```python
from build123d import *

# Parameters (mm, degrees)
F0_R     = 20
F1_DEPTH = 3.5
F3_R     = 20
F4_DEPTH = 2
F5_W     = 55
F5_H     = 9.110272
F6_DEPTH = 2


with BuildPart() as f1:
    # F0 (on Top) → F1 (new body)
    with BuildSketch(Plane.XY):
        Circle(F0_R)
        Polygon((-12.444864, 12.444864), (-4.555136, 17), (4.555136, 17), (12.444864, 12.444864), (17, 4.555136), (17, -4.555136), (12.444864, -12.444864), (4.555136, -17), (-4.555136, -17), (-12.444864, -12.444864), (-17, -4.555136), (-17, 4.555136), align=None, mode=Mode.SUBTRACT)
    extrude(amount=F1_DEPTH)

    # F3 (on Top) → F4 (join)
    with BuildSketch(Plane.XY):
        Circle(F3_R)
    extrude(amount=F4_DEPTH)

    # F5 (on Top) → F6 (join)
    with BuildSketch(Plane.XY):
        Rectangle(F5_W, F5_H)
    extrude(amount=F6_DEPTH)


solid = f1.part
```
The listing builds one solid part. Answer for the finished solid, in the listing's coordinates (mm). A direction names the side the tool comes from. Give positions to 0.01 mm unless a question says otherwise; leave off trailing zeros. Write each loop counter-clockwise with the first axis right and the second up, starting at its lowest first coordinate (ties: lowest second). Pieces come first, ordered by that corner, then holes. Notation, with made-up numbers: (-3.75, 31) - (2.25, 31) arc R16 ccw to (2.25, 56) - close; hole circle Ø10 at (8.25, 74). An arc over 180 degrees is marked (long way). Use one line per item in the form item = value. Start each with the question number.
1) A tool of negligible diameter and unlimited length cuts with its end or side. For faces 1 (the face through (0, 17, 3)), 2 (the face through (23, 4.555, 1)), 3 (the face through (-27.5, 0, 1)), 4 (the face through (0, 0, 0)), 5 (the face through (-24, -4.555, 1)), from which of +Z, -Z, +X, -X, +Y, -Y can it reach the whole face along a straight path? Write none if from no direction.
2) Consider line 1 along Y through (x, z) = (-0.5, 3); line 2 along Z through (x, y) = (-21.5, 3.5); line 3 along Y through (x, z) = (-15, 2.3). Determine where each line is inside the solid, lowest interval first. Write a range as from..to.
3) Find section C-C on x = 0. Determine the outline of the cut face in (y, z).
4) Find section B-B on y = 0. Determine the outline of the cut face in (x, z), plus the area to 3 significant figures.
5) Flat-ended cylindrical pins translate along their axes: pin 1 Ø1.2 at (y, z) = (0, 2.5) entering from -X; pin 2 Ø2 at (x, z) = (24.5, 1.5) entering from -Y; pin 3 Ø1.6 at (x, z) = (22, 1) entering from +Y; pin 4 Ø17 at (x, y) = (-7, 0.5) entering from +Z. Find the tip coordinate at first contact, or state that the pin passes through.
6) Find section D-D on y = 8. Determine the outline of the cut face in (x, z).
7) Find section A-A on z = 2.85. Determine the outline of the cut face in (x, y).
8) The mould has two halves that part along Y. Classify faces 6 (the face through (-24, 4.555, 1)), 7 (the face through (23, -4.555, 1)), 8 (the face through (14.69, 8.56, 2.74)): pulls with the +Y half, pulls with the -Y half, needs draft (parallel to the pull), parting line crosses it, or undercut.
Geometry results:
q1.face_1 = +Z
q1.face_2 = +Z, -Z, +X, +Y
q1.face_3 = +Z, -Z, -X, +Y, -Y
q1.face_4 = -Z, +X, -X, +Y, -Y
q1.face_5 = +Z, -Z, -X, -Y
q2.line_1 = -19.99..-17, 17..19.99
q2.line_2 = 0..2
q2.line_3 = -13.23..-8.02, 8.02..13.23
q3.outline = (-20, 0) - (20, 0) - (20, 3.5) - (17, 3.5) - (17, 2) - (-17, 2) - (-17, 3.5) - (-20, 3.5) - close
q4.outline = (-27.5, 0) - (27.5, 0) - (27.5, 2) - (20, 2) - (20, 3.5) - (17, 3.5) - (17, 2) - (-17, 2) - (-17, 3.5) - (-20, 3.5) - (-20, 2) - (-27.5, 2) - close
q4.area = 119 mm2
q5.pin_1 = -27.5
q5.pin_2 = -4.56
q5.pin_3 = 4.56
q5.pin_4 = 2
q6.outline = (-18.33, 0) - (18.33, 0) - (18.33, 3.5) - (15.01, 3.5) - (15.01, 2) - (-15.01, 2) - (-15.01, 3.5) - (-18.33, 3.5) - close
q7.outline = circle Ø40 at (0, 0); hole (-17, -4.56) - (-12.44, -12.44) - (-4.56, -17) - (4.56, -17) - (12.44, -12.44) - (17, -4.56) - (17, 4.56) - (12.44, 12.44) - (4.56, 17) - (-4.56, 17) - (-12.44, 12.44) - (-17, 4.56) - close
q8.face_6 = pulls with the +Y half
q8.face_7 = pulls with the -Y half
q8.face_8 = undercut
